Check sheet for the modelled part. Datum: model origin and axes. Units: mm. A direction names the side the tool comes from. Give positions to 0.01 mm unless a question says otherwise; leave off trailing zeros. Loops run counter-clockwise (first coordinate to the right, second up) from the corner with the lowest first, then second, coordinate; pieces in that order, holes last. Notation, with made-up numbers: (29.25, 45.5) - (51.25, 45.5) arc R25 cw to (51.25, 62.5) - close; hole circle Ø11 at (13.5, 51). An arc over 180 degrees is marked (long way). Answer in a Markdown table with one row per item. Add a question column.
(1) Go/stop test with flat-tipped pins: P1, Ø3, axis at x = 44.45, z = 21.11, coming from the -Y side; P2, Ø1.5, axis at x = 54.5, y = 1, coming from the -Z side; P3, Ø4, axis at x = 44.45, z = -14.45, coming from the +Y side; P4, Ø1.9, axis at y = 4, z = -8.5, coming from the +X side. Record where each tip stops, or that it passes through.
(2) Sectioned sample at D-D on y = 4.5. State how many separate pieces and enclosed holes the cut face has, then the cut area to 3 significant figures.
(3) Set-up check for faces 4 (the face through (44, 3, -23.34)), 5 (the face through (54.61, 3, -6)), 6 (the face through (54.61, 3, 48)), 7 (the face through (17, 3, 31.27)): record each of +Z, -Z, +X, -X, +Y, -Y from which the full face is reachable in a straight line by a thin tool's end or side.
(4) Draft check along X on faces 1 (the face through (36.581, 3.219, -21.167)), 2 (the face through (38, 6.35, 21)), 3 (the face through (46.398, 3.131, -14.705)). Enter one of: released by +X, released by -X, zero draft, split by the parting line, or undercut.
(5) Sectioned sample at C-C on z = 43. Enter the section's corners in (x, y).
(6) Sectioned sample at B-B on x = 80.01. Enter the section's corners in (y, z).
(7) Sectioned sample at A-A on x = 44.45. Enter the section's corners in (y, z).
(8) Thickness scan on L1, parallel to Z at x = 44.45, y = 1.7; L2, parallel to Z at x = 47, y = 5 (1 decimal); L3, parallel to Z at x = 8.89, y = 0.8. Record the ranges inside material, lowest first.
Autodesk Inventor part; units mm, degrees
ref_plane "YZ Plane" through (0, 0, 0) normal (1, 0, 0) x (0, 1, 0)
ref_plane "XZ Plane" through (0, 0, 0) normal (0, 1, 0) x (-1, 0, 0)
ref_plane "XY Plane" through (0, 0, 0) normal (0, 0, 1) x (1, 0, 0)
sketch "Sketch1" plane through (0, 0, 0) normal (0, 1, 0) x (-1, 0, 0)
  line L0 (0, -23.3395) -> (-88.9, -23.3395)
  line L1 (-88.9, -23.3395) -> (-88.9, 65.5605)
  line L2 (-88.9, 65.5605) -> (0, 65.5605)
  line L3 (0, 65.5605) -> (0, -23.3395)
  point P0 (0, 0)
  dimension "d0" = 88.9
  dimension "d1" = 88.9
extrude "Extrusion1" add sketch "Sketch1" along normal blind 6.35
sketch "Sketch2" plane through (0, 6.35, 0) normal (0, 1, 0) x (1, 0, 0)
  line L0 (88.9, -65.5605) -> (88.9, 23.3395)
  line L1 (88.9, 23.3395) -> (0, 23.3395)
  point P0 (0, 0)
  point P1 (44.45, -21.1105)
  point P2 (80.01, -21.1105)
  point P3 (8.89, -21.1105)
  point P4 (44.45, 14.4495)
  point P5 (44.45, -56.6705)
  dimension "d4" = 44.45
  dimension "d5" = 44.45
  dimension "d6" = 35.56
  dimension "d7" = 35.56
  dimension "d8" = 35.56
  dimension "d9" = 35.56
hole "Hole1" at (44.45, 6.35, 21.1105) at (80.01, 6.35, 21.1105) at (8.89, 6.35, 21.1105) at (44.45, 6.35, -14.4495) at (44.45, 6.35, 56.6705) direction (0, -1, 0) diameter 3.556 end through all countersink diameter 9.525 countersink angle 82
sketch "Sketch3" plane through (0, 6.35, 0) normal (0, 1, 0) x (1, 0, 0)
  line L0 (88.9, 23.3395) -> (0, 23.3395)
  line L1 (88.9, -65.5605) -> (0, -65.5605)
  line L2 (0, -65.5605) -> (0, 23.3395)
  line L3 (88.9, 23.3395) -> (88.9, -65.5605)
  line L4 (34.29, 15.7195) -> (34.29, -3.3305)
  line L5 (34.29, -38.8905) -> (34.29, -57.9405)
  line L6 (54.61, 15.7195) -> (54.61, -3.3305)
  line L7 (54.61, -38.8905) -> (54.61, -57.9405)
  line L8 (7.62, -31.2705) -> (26.67, -31.2705)
  line L9 (62.23, -31.2705) -> (81.28, -31.2705)
  line L10 (7.62, -10.9505) -> (26.67, -10.9505)
  line L11 (62.23, -10.9505) -> (81.28, -10.9505)
  line L12 (0, -18.5705) -> (0, -23.6505)
  line L13 (41.91, -65.5605) -> (46.99, -65.5605)
  line L14 (88.9, -23.6505) -> (88.9, -18.5705)
  line L15 (41.91, 23.3395) -> (46.99, 23.3395)
  arc A0 (41.91, 23.3395) -> (34.29, 15.7195) centre (41.91, 15.7195) ccw
  arc A1 (54.61, 15.7195) -> (46.99, 23.3395) centre (46.99, 15.7195) ccw
  arc A2 (26.67, -10.9505) -> (34.29, -3.3305) centre (26.67, -3.3305) ccw
  arc A3 (7.62, -10.9505) -> (0, -18.5705) centre (7.62, -18.5705) ccw
  arc A4 (0, -23.6505) -> (7.62, -31.2705) centre (7.62, -23.6505) ccw
  arc A5 (34.29, -38.8905) -> (26.67, -31.2705) centre (26.67, -38.8905) ccw
  arc A6 (34.29, -57.9405) -> (41.91, -65.5605) centre (41.91, -57.9405) ccw
  arc A7 (46.99, -65.5605) -> (54.61, -57.9405) centre (46.99, -57.9405) ccw
  arc A8 (62.23, -31.2705) -> (54.61, -38.8905) centre (62.23, -38.8905) ccw
  arc A9 (81.28, -31.2705) -> (88.9, -23.6505) centre (81.28, -23.6505) ccw
  arc A10 (88.9, -18.5705) -> (81.28, -10.9505) centre (81.28, -18.5705) ccw
  arc A11 (54.61, -3.3305) -> (62.23, -10.9505) centre (62.23, -3.3305) ccw
  point P0 (0, 0)
  dimension "d21" = 7.62
extrude "Extrusion2" cut sketch "Sketch3" against normal blind 6.35 contours L3 A10 L11 A11 L6 A1 L0 | A0 L4 A2 L10 A3 L2 L0 | L3 L1 A7 L7 A8 L9 A9 | A4 L8 A5 L5 A6 L1 L2
properties part number "plus sign" material "Polypropylene"
Reply:
| question | item | result |
|---|---|---|
| 1 | P1 | through |
| 1 | P2 | z = -19.24 |
| 1 | P3 | y = 3.17 |
| 1 | P4 | x = 54.61 |
| 2 | separate pieces | 1 |
| 2 | enclosed holes | 5 |
| 2 | area | 2,990 mm^2 |
| 3 | face 4 | -Z, +X, -X, +Y, -Y |
| 3 | face 5 | -Z, +X, +Y, -Y |
| 3 | face 6 | +Z, +X, +Y, -Y |
| 3 | face 7 | +Z, -X, +Y, -Y |
| 4 | face 1 | released by -X |
| 4 | face 2 | zero draft |
| 4 | face 3 | undercut |
| 5 | outline | (34.29, 0) - (54.61, 0) - (54.61, 6.35) - (34.29, 6.35) - close |
| 6 | outline | (0, 10.95) - (6.35, 10.95) - (6.35, 16.35) - (2.92, 19.33) - (0, 19.33) - close; (0, 22.89) - (2.92, 22.89) - (6.35, 25.87) - (6.35, 31.27) - (0, 31.27) - close |
| 7 | outline | (0, -23.34) - (6.35, -23.34) - (6.35, -19.21) - (2.92, -16.23) - (0, -16.23) - close; (0, -12.67) - (2.92, -12.67) - (6.35, -9.69) - (6.35, 16.35) - (2.92, 19.33) - (0, 19.33) - close; (0, 22.89) - (2.92, 22.89) - (6.35, 25.87) - (6.35, 51.91) - (2.92, 54.89) - (0, 54.89) - close; (0, 58.45) - (2.92, 58.45) - (6.35, 61.43) - (6.35, 65.56) - (0, 65.56) - close |
| 8 | L1 | -23.34 to -16.23, -12.67 to 19.33, 22.89 to 54.89, 58.45 to 65.56 |
| 8 | L2 | -23.3 to -17, -11.9 to 18.6, 23.6 to 54.1, 59.2 to 65.6 |
| 8 | L3 | 10.95 to 19.33, 22.89 to 31.27 |
